Geometry: final body of the model. Coordinates: model frame, mm. Face numbers are marked on the shaded views. A direction names the side the tool comes from. Give positions to 0.01 mm unless a question says otherwise; leave off trailing zeros. Loops run counter-clockwise (first coordinate to the right, second up) from the corner with the lowest first, then second, coordinate; pieces in that order, holes last. Notation, with made-up numbers: (-5, 8.25) -> (2, 8.25) arc R27 ccw to (2, 26.25) -> close; hole circle Ø3 at (80.5, 57.5). An arc over 180 degrees is marked (long way). Answer in a Markdown table with one row per item. Add a question column.
1) First-contact query: P1, Ø3, axis at y = 11, z = -1, coming from the -X side; P2, Ø1, axis at y = 0, z = -1, coming from the -X side; P3, Ø2.5, axis at y = 2, z = -0.5, coming from the +X side; P4, Ø1, axis at x = -5, z = -2.5, coming from the +Y side. Flat tips, straight axial feed; report the tip coordinate or a pass-through.
2) Section query D-D (y = 10.5). Return the cut outline in (x, z).
3) Draft query along Z for the marked faces 1, 2 and 3. Return one class per face: +Z half, -Z half, draft (parallel to the pull), parting line (faces both ways), or undercut.
4) Access query for the marked faces 4, 5 and 6. Directions: +Z, -Z, +X, -X, +Y, -Y. A direction counts if a zero-diameter tool reaches every point of the face in a straight line with its end or side. Return the directions, or none.
5) Line query: line 1 (Z direction, x = -6.5, y = -9.5); line 2 (Y direction, x = -3, z = 2); line 3 (X direction, y = -11.25, z = -2). Output: solid intervals per line, ascending. Write a range as from..to.
6) Section query A-A (y = -1). Return the cut outline in (x, z).
7) Section query B-B (x = -3.75). Return the cut outline in (y, z).
8) Section query C-C (x = -6). Return the cut outline in (y, z).
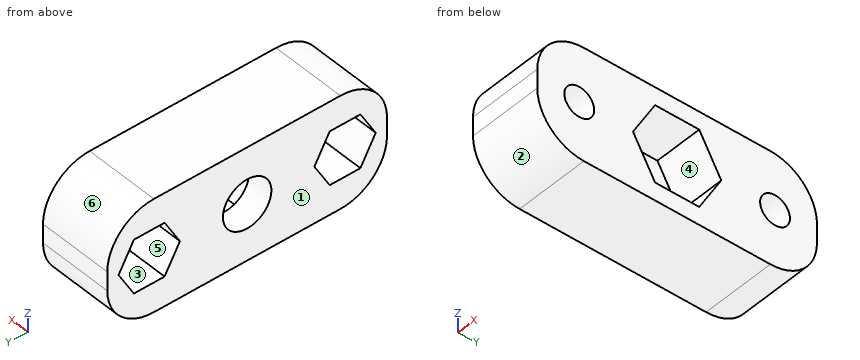
```python
from build123d import *

# Parameters (mm, degrees)
SKIZZE1_W                       = 8
SKIZZE1_H                       = 30
AUFSATZ_LINEAR_AUSTRAGEN1_DEPTH = 6
SCHNITT_LINEAR_AUSTRAGEN3_DEPTH = 5.2
SCHNITT_LINEAR_START            = -8
SCHNITT_LINEAR_AUSTRAGEN2_DEPTH = 5.2
SKIZZE4_R                       = 1.6
SKIZZE4_R_2                     = 2.6
SCHNITT_LINEAR_AUSTRAGEN4_DEPTH = 19.027756377
VERRUNDUNG1_R                   = 5


with BuildPart() as part:
    # Skizze1 → Aufsatz-Linear austragen1 (new, symmetric)
    with BuildSketch(Plane.XY):
        with Locations((-4, 0)):
            Rectangle(SKIZZE1_W, SKIZZE1_H)
    extrude(amount=AUFSATZ_LINEAR_AUSTRAGEN1_DEPTH, both=True)

    # Skizze2 → Schnitt-Linear austragen3 (cut)
    with BuildSketch(Plane(origin=(0, 0, 0), x_dir=(0, 0, -1), z_dir=(1, 0, 0))):
        Polygon((0, 4.734272207), (-4.1, 2.367136104), (-4.1, -2.367136104), (0, -4.734272207), (4.1, -2.367136104), (4.1, 2.367136104), align=None)
    extrude(amount=-SCHNITT_LINEAR_AUSTRAGEN3_DEPTH, mode=Mode.SUBTRACT)

    # Skizze3 → Schnitt-Linear austragen2 (cut)
    with BuildSketch(Plane(origin=(0, 0, 0), x_dir=(0, 0, -1), z_dir=(1, 0, 0)).offset(SCHNITT_LINEAR_START)):
        Polygon((2.85, 8.854551733), (2.85, 12.145448267), (0, 13.790896534), (-2.85, 12.145448267), (-2.85, 8.854551733), (0, 7.209103466), align=None)
    schnitt_linear_austragen2 = extrude(amount=SCHNITT_LINEAR_AUSTRAGEN2_DEPTH, mode=Mode.SUBTRACT)

    # Skizze4 → Schnitt-Linear austragen4 (cut, through all)
    with BuildSketch(Plane(origin=(0, 0, 0), x_dir=(0, 0, -1), z_dir=(1, 0, 0))):
        with Locations((0, 10.5)):
            Circle(SKIZZE4_R)
        with Locations((0, -10.5)):
            Circle(SKIZZE4_R)
        Circle(SKIZZE4_R_2)
    extrude(amount=-SCHNITT_LINEAR_AUSTRAGEN4_DEPTH, mode=Mode.SUBTRACT)

    # Spiegeln1: Schnitt-Linear austragen2 across plane
    add(schnitt_linear_austragen2.mirror(Plane.ZX), mode=Mode.SUBTRACT)

    # Verrundung1
    verrundung1_edges = [part.edges().sort_by_distance(p)[0] for p in [
        (-4, -15, 6),
        (-4, -15, -6),
        (-4, 15, -6),
        (-4, 15, 6),
    ]]
    fillet(verrundung1_edges, radius=VERRUNDUNG1_R)


solid = part.part
```
Evaluation:
| question | item | result |
|---|---|---|
| 1 | P1 | x = -2.8 |
| 1 | P2 | through |
| 1 | P3 | x = -5.2 |
| 1 | P4 | y = 14.9 |
| 2 | outline | (-8, -5.97) -> (0, -5.97) -> (0, -1.6) -> (-2.8, -1.6) -> (-2.8, -2.85) -> (-8, -2.85) -> close; (-8, 2.85) -> (-2.8, 2.85) -> (-2.8, 1.6) -> (0, 1.6) -> (0, 5.97) -> (-8, 5.97) -> close |
| 3 | face 1 | draft |
| 3 | face 2 | -Z half |
| 3 | face 3 | undercut |
| 4 | face 4 | +X |
| 4 | face 5 | -X |
| 4 | face 6 | +Z, +X, -X, +Y |
| 5 | line 1 | -6..-2.85, 2.85..6 |
| 5 | line 2 | -14.9..-12.64, -8.36..-3.58, 3.58..8.36, 12.64..14.9 |
| 5 | line 3 | -2.8..0 |
| 6 | outline | (-8, -6) -> (0, -6) -> (0, -4.1) -> (-5.2, -4.1) -> (-5.2, -2.4) -> (-8, -2.4) -> close; (-8, 2.4) -> (-5.2, 2.4) -> (-5.2, 4.1) -> (0, 4.1) -> (0, 6) -> (-8, 6) -> close |
| 7 | outline | (-15, -1) arc R5 ccw to (-10, -6) -> (10, -6) arc R5 ccw to (15, -1) -> (15, 1) arc R5 ccw to (10, 6) -> (-10, 6) arc R5 ccw to (-15, 1) -> close; hole (-13.79, 0) -> (-12.15, -2.85) -> (-8.85, -2.85) -> (-7.21, 0) -> (-8.85, 2.85) -> (-12.15, 2.85) -> close; hole (-4.73, 0) -> (-2.37, -4.1) -> (2.37, -4.1) -> (4.73, 0) -> (2.37, 4.1) -> (-2.37, 4.1) -> close; hole (7.21, 0) -> (8.85, -2.85) -> (12.15, -2.85) -> (13.79, 0) -> (12.15, 2.85) -> (8.85, 2.85) -> close |
| 8 | outline | (-15, -1) arc R5 ccw to (-10, -6) -> (10, -6) arc R5 ccw to (15, -1) -> (15, 1) arc R5 ccw to (10, 6) -> (-10, 6) arc R5 ccw to (-15, 1) -> close; hole (-13.79, 0) -> (-12.15, -2.85) -> (-8.85, -2.85) -> (-7.21, 0) -> (-8.85, 2.85) -> (-12.15, 2.85) -> close; hole circle Ø5.2 at (0, 0); hole (7.21, 0) -> (8.85, -2.85) -> (12.15, -2.85) -> (13.79, 0) -> (12.15, 2.85) -> (8.85, 2.85) -> close |
